Here's how the part is built. I have some questions about the finished solid (model axes, mm). A direction names the side the tool comes from. Coordinates: 2 decimals unless noted, no trailing zeros. Order: outer loops, then holes, each group sorted by start corner. A loop starts at its lowest first (then second) coordinate and runs counter-clockwise, first axis right, second up. Notation, with made-up numbers: M -9,3 L 45,3 A20 cw 45,7 Z; hole C 35.25,-2 d1. An arc over 180 degrees is marked long. Answer as CSV lines item,"result". Start each with the question number.
```python
from build123d import *

# Parameters (mm, degrees)
SKETCH1_R           = 4.5000037
BOSS_EXTRUDE1_DEPTH = 3.75000012
SKETCH2_R           = 4.5000037
SKETCH2_R_2         = 3.499999998
SKETCH2_R_3         = 1.25000004
BOSS_EXTRUDE2_DEPTH = 1.750000056
SKETCH4_R           = 2.75000466
SKETCH4_R_2         = 1.25000004
CUT_EXTRUDE1_DEPTH  = 0.875000028
SKETCH6_R           = 4.5000037
SKETCH6_R_2         = 3.5000057
CUT_EXTRUDE2_DEPTH  = 0.875000028
SKETCH7_R           = 10.5000044
SKETCH7_R_2         = 4.5000037
BOSS_EXTRUDE3_DEPTH = 1.750000056
SKETCH9_R           = 0.62500002
CUT_EXTRUDE3_DEPTH  = 6.500000176
CIRPATTERN1_COUNT   = 4
CHAMFER1_SIZE       = 0.999998
CHAMFER1_SIZE2      = 0.577349114


with BuildPart() as part:
    # Sketch1 → Boss-Extrude1 (new body)
    with BuildSketch(Plane.XY):
        with Locations((-10.24995918, 0)):
            Circle(SKETCH1_R)
        Polygon((-10.24995918, 2.999994), (-10.594624819, 2.728309468), (-10.996027349, 2.905743672), (-11.262299488, 2.55687975), (-11.695217312, 2.628914782), (-11.866365092, 2.224791874), (-12.303596391, 2.186901508), (-12.368865968, 1.752912142), (-12.782937891, 1.60747717), (-12.738228138, 1.170890494), (-13.103123023, 0.927049129), (-12.951243218, 0.515297489), (-13.244033377, 0.188371182), (-12.994526687, -0.172673551), (-13.196815038, -0.562142819), (-12.865358886, -0.849794878), (-12.964434908, -1.27733532), (-12.571855902, -1.473520467), (-12.561494285, -1.912268145), (-12.132459609, -2.004659346), (-12.01331141, -2.427046129), (-11.574778889, -2.409838105), (-11.354330629, -2.789323879), (-10.933854876, -2.663597874), (-10.625958129, -2.976338151), (-10.24995918, -2.749993992), (-9.873960231, -2.976338151), (-9.566063484, -2.663597874), (-9.145587731, -2.789323879), (-8.925139471, -2.409838105), (-8.48660695, -2.427046129), (-8.367458751, -2.004659346), (-7.938424075, -1.912268145), (-7.928062458, -1.473520467), (-7.535483452, -1.27733532), (-7.634559474, -0.849794878), (-7.303103322, -0.562142819), (-7.505391673, -0.172673551), (-7.255884983, 0.188371182), (-7.548675142, 0.515297489), (-7.396795337, 0.927049129), (-7.761690222, 1.170890494), (-7.716980469, 1.60747717), (-8.131052392, 1.752912142), (-8.196321969, 2.186901508), (-8.633553268, 2.224791874), (-8.804701048, 2.628914782), (-9.237618872, 2.55687975), (-9.503891011, 2.905743672), (-9.905293541, 2.728309468), align=None, mode=Mode.SUBTRACT)
    extrude(amount=-BOSS_EXTRUDE1_DEPTH)

    # Sketch2 → Boss-Extrude2 (add)
    with BuildSketch(Plane.XY):
        with Locations((-10.24995918, 0)):
            Circle(SKETCH2_R)
        with Locations((-10.24995918, 0)):
            Circle(SKETCH2_R_2, mode=Mode.SUBTRACT)
        with Locations((-10.24995918, 0)):
            Circle(SKETCH2_R_2)
        with Locations((-10.24995918, 0)):
            Circle(SKETCH2_R_3, mode=Mode.SUBTRACT)
    extrude(amount=BOSS_EXTRUDE2_DEPTH)

    # Sketch4 → Cut-Extrude1 (cut)
    with BuildSketch(Plane.XY.offset(1.750000056)):
        with Locations((-10.24995918, 0)):
            Circle(SKETCH4_R)
        with Locations((-10.24995918, 0)):
            Circle(SKETCH4_R_2, mode=Mode.SUBTRACT)
    extrude(amount=-CUT_EXTRUDE1_DEPTH, mode=Mode.SUBTRACT)

    # Sketch6 → Cut-Extrude2 (cut)
    with BuildSketch(Plane.XY.offset(1.750000056)):
        with Locations((-10.24995918, 0)):
            Circle(SKETCH6_R)
        with Locations((-10.24995918, 0)):
            Circle(SKETCH6_R_2, mode=Mode.SUBTRACT)
    extrude(amount=-CUT_EXTRUDE2_DEPTH, mode=Mode.SUBTRACT)

    # Sketch7 → Boss-Extrude3 (add)
    with BuildSketch(Plane.XY.offset(1.750000056)):
        with Locations((-10.24995918, 0)):
            Circle(SKETCH7_R)
        with Locations((-10.24995918, 0)):
            Circle(SKETCH7_R_2, mode=Mode.SUBTRACT)
    extrude(amount=-BOSS_EXTRUDE3_DEPTH)

    # Sketch9 → Cut-Extrude3 (cut, through all)
    with BuildSketch(Plane.XY.offset(1.750000056)):
        with Locations((-10.24995918, 7.8750033)):
            Circle(SKETCH9_R)
        with Locations((-14.124959304, 7.8750033)):
            Circle(SKETCH9_R)
        with Locations((-6.374959056, 7.8750033)):
            Circle(SKETCH9_R)
    cut_extrude3 = extrude(amount=-CUT_EXTRUDE3_DEPTH, mode=Mode.SUBTRACT)

    # CirPattern1: Cut-Extrude3 ×4 about axis
    cirpattern1_axis = Axis((-10.24995918, 0, 0), (0, 0, 1))
    for i in range(1, CIRPATTERN1_COUNT):
        add(cut_extrude3.rotate(cirpattern1_axis, i * 360 / CIRPATTERN1_COUNT), mode=Mode.SUBTRACT)

    # Chamfer1
    chamfer1_edges = [part.edges().sort_by_distance(p)[0] for p in [
        (-14.74996288, 0, 0),
    ]]
    chamfer1_side = [part.faces().sort_by_distance(p)[0] for p in [
        (-14.74996288, 0, -1.87500006),
    ]]
    chamfer(chamfer1_edges, length=CHAMFER1_SIZE, length2=CHAMFER1_SIZE2, reference=chamfer1_side[0])


solid = part.part
```
1) If we mould it in two halves opening along X, with no side actions, what happens to faces 4 (the face through (-9.095, -0.479, 0.431)), 5 (the face through (-7, 0, -3.75)), 6 (the face through (-18.58, -6.39, 0.89))? For each: released by +X, released by -X, zero draft, split by the parting line, or undercut.
2) Which directions (+Z, -Z, +X, -X, +Y, -Y) give clear straight access to the entire face, cutting with the end or side of a thin tool? Please do faces 1 (the face through (-13, -5, 0)), 2 (the face through (-2.755, -3.379, 0.887)), 3 (the face through (-5.958, 1.352, 1.319)).
3) Suppose I cut it at D-D on x = -16.5. Please give me the cut outline in (y, z).
4) Suppose I cut it at A-A on z = 0.3. Give the number of separate pieces and of enclosed holes in the cut face, plus the area to 3 significant figures.
5) I need wall thicknesses on line 1 (Y direction, x = -18, z = 0.4); line 2 (Z direction, x = -14.75, y = -7.25); line 3 (Y direction, x = -11.25, z = -0.6). Which ranges of each line are inside material? Lowest first, please. Write a range as [from, to].
6) Will these pins go through, and if not, where does the flat tip stop? pin 1 Ø3 at (x, y) = (-17, 5.5) entering from -Z; pin 2 Ø3 at (x, z) = (-4, 1) entering from -Y; pin 3 Ø1 at (x, y) = (-13.5, -4) entering from -Z.
Output:
1,face 4,"undercut"
1,face 5,"zero draft"
1,face 6,"split by the parting line"
2,face 1,"-Z"
2,face 2,"+Z, -Z"
2,face 3,"+Z"
3,outline,"M -8.44,0 L 8.44,0 L 8.44,1.75 L -8.44,1.75 Z"
4,separate pieces,"1"
4,enclosed holes,"13"
4,area,"327 mm²"
5,line 1,"[-7.08, -4.49], [-3.26, -0.61], [0.61, 3.26], [4.49, 7.08]"
5,line 2,"[0, 1.75]"
5,line 3,"[-4.62, -2.76], [2.57, 4.62]"
6,pin 1,"z = 0"
6,pin 2,"y = -9.36"
6,pin 3,"z = -0.73"
